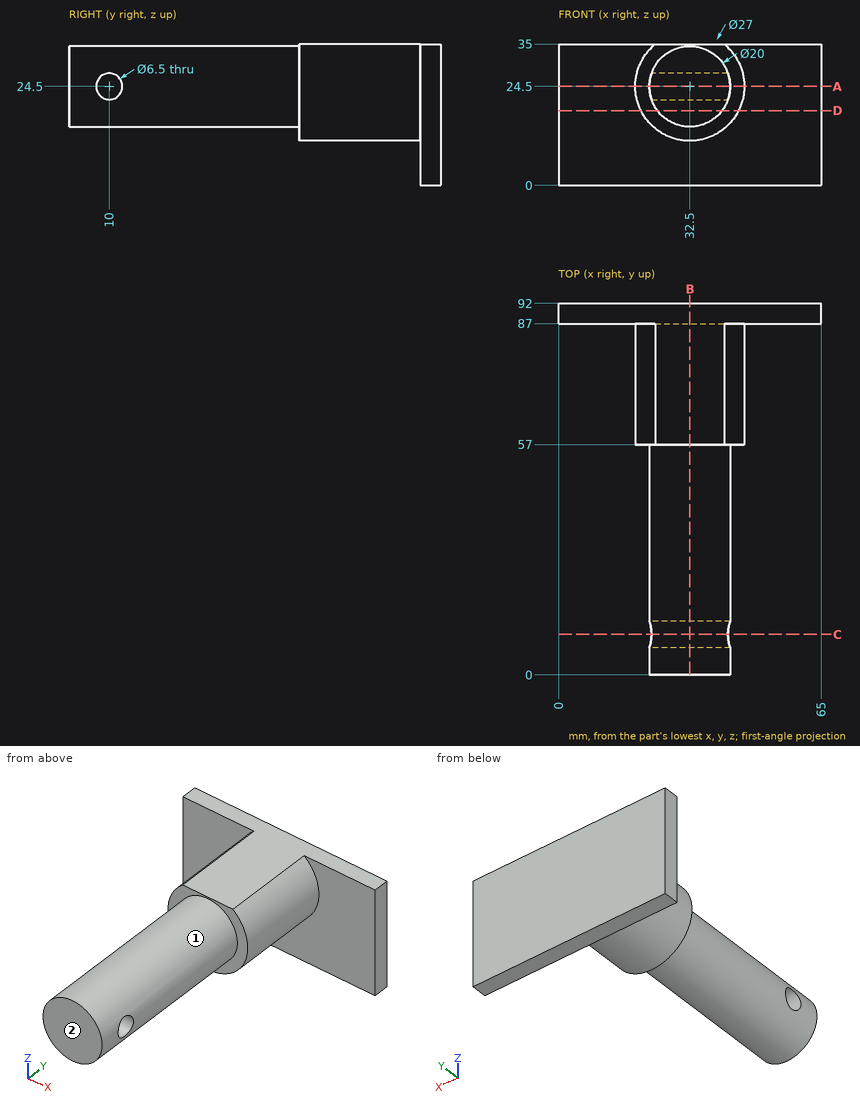
Could you check a few things on this drawing? It's one solid part, dimensions in mm from its lowest x, y, z. A direction names the side the tool comes from. Round coordinates to 2 decimals unless told otherwise and drop trailing zeros. Write each loop counter-clockwise with the first axis right and the second up, starting at its lowest first coordinate (ties: lowest second). Pieces come first, ordered by that corner, then holes. Notation, with made-up numbers: (86, 32) -> (90, 32) arc R12 ccw to (90, 55) -> close; hole circle Ø8 at (-21, -30.75). An arc over 180 degrees is marked (long way). Use a Markdown table: item, result.
1. Which directions (+Z, -Z, +X, -X, +Y, -Y) give clear straight access to the entire face, cutting with the end or side of a thin tool? Please do the marked faces 1 and 2.
Answer key:
| item | result |
|---|---|
| face 1 | -Y |
| face 2 | +Z, -Z, +X, -X, -Y |
2. If we section it at B-B (x = 32.5): List the corners of the cut face in (y, z) for me, then the cut area to 3 significant figures.
Answer key:
| item | result |
|---|---|
| outline | (0, 14.5) -> (57, 14.5) -> (57, 11) -> (87, 11) -> (87, 0) -> (92, 0) -> (92, 35) -> (57, 35) -> (57, 34.5) -> (0, 34.5) -> close; hole circle Ø6.5 at (10, 24.5) |
| area | 2,000 mm^2 |
3. For pin 1 Ø10 at (x, y) = (51.5, 17.5) entering from -Z; pin 2 Ø8 at (y, z) = (12.5, 21) entering from -X; pin 3 Ø8 at (y, z) = (61.5, 17.5) entering from +X, each with a flat end and sliding along its axis, tell me the tip position at first contact or that it passes through.
Answer key:
| item | result |
|---|---|
| pin 1 | passes through |
| pin 2 | stops at x = 22.5 |
| pin 3 | stops at x = 45.66 |
4. If we section it at D-D (z = 18.5): List the corners of the cut face in (x, y) for me.
Answer key:
| item | result |
|---|---|
| outline | (0, 87) -> (20.41, 87) -> (20.41, 57) -> (24.5, 57) -> (24.5, 0) -> (40.5, 0) -> (40.5, 57) -> (44.59, 57) -> (44.59, 87) -> (65, 87) -> (65, 92) -> (0, 92) -> close |
5. Please list where these lines run through material, in increasing order: probe 1 along Y at (x, z) = (32.5, 24.5); probe 2 along Y at (x, z) = (12, 32); probe 3 along Y at (x, z) = (32.5, 23.5).
Answer key:
| item | result |
|---|---|
| probe 1 | y = 0 to 6.75, 13.25 to 92 |
| probe 2 | y = 87 to 92 |
| probe 3 | y = 0 to 6.91, 13.09 to 92 |
6. If we section it at A-A (z = 24.5): List the corners of the cut face in (x, y) for me, then the cut area to 4 significant figures.
Answer key:
| item | result |
|---|---|
| outline | (0, 87) -> (19, 87) -> (19, 57) -> (22.5, 57) -> (22.5, 13.25) -> (42.5, 13.25) -> (42.5, 57) -> (46, 57) -> (46, 87) -> (65, 87) -> (65, 92) -> (0, 92) -> close; (22.5, 0) -> (42.5, 0) -> (42.5, 6.75) -> (22.5, 6.75) -> close |
| area | 2,145 mm^2 |
7. If we section it at C-C (y = 10): List the corners of the cut face in (x, z) for me.
Answer key:
| item | result |
|---|---|
| outline | (23.04, 21.25) arc R10 ccw to (41.96, 21.25) -> close; (23.04, 27.75) -> (41.96, 27.75) arc R10 ccw to start |
